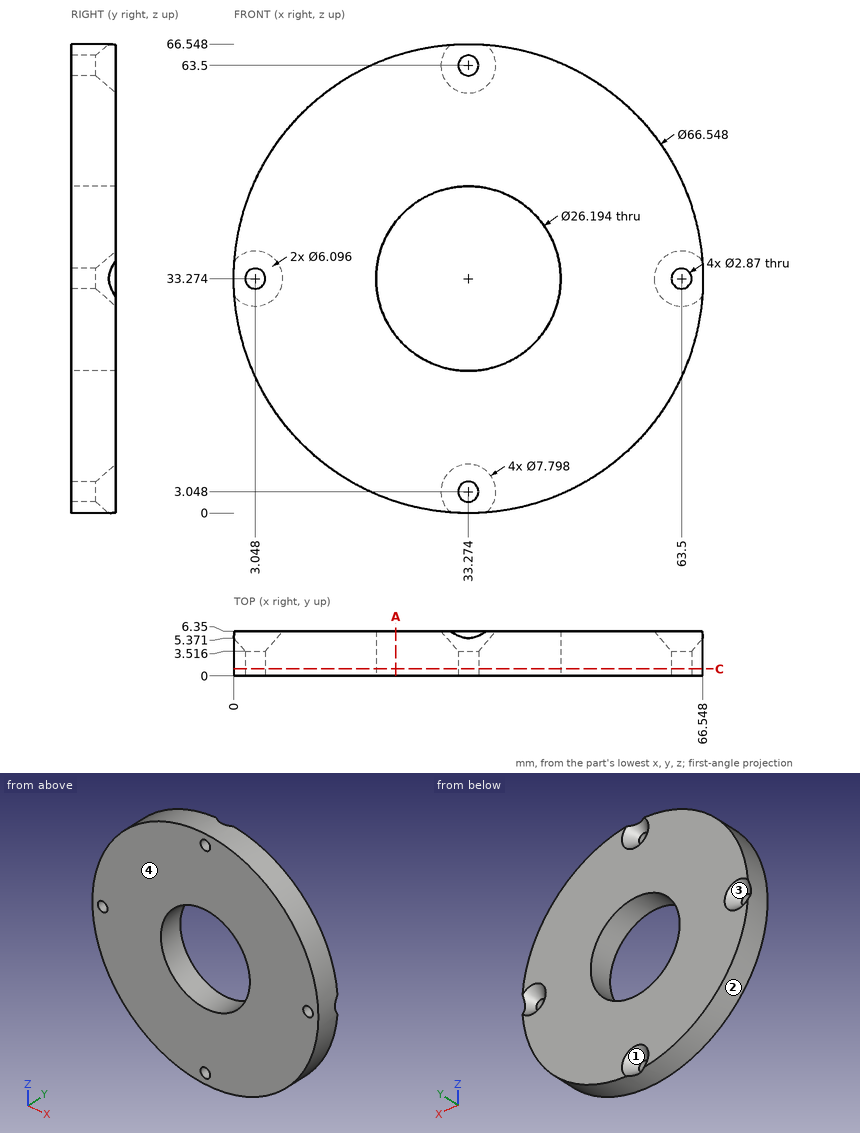
Check sheet for the drawn part. Datum: minimum x, y, z corner. Units: mm. Coordinates: 2 decimals unless noted, no trailing zeros. Write each loop counter-clockwise with the first axis right and the second up, starting at its lowest first coordinate (ties: lowest second). Pieces come first, ordered by that corner, then holes. Notation, with made-up numbers: (21, 62) - (63, 62) arc R33 cw to (63, 95) - close; hole circle Ø9 at (-36, 47.5). An arc over 180 degrees is marked (long way). Answer as a JSON object with one key per item and string values.
(1) Mould release check, pull along Z, two halves, no side actions. Record for the marked faces 1, 2, 3 and 4: pulls with the +Z half, pulls with the -Z half, needs draft (parallel to the pull), parting line crosses it, or undercut.
Report:
{"face 1": "undercut", "face 2": "parting line crosses it", "face 3": "undercut", "face 4": "needs draft"}
(2) Thickness scan on line 1 along Z through (x, y) = (34.5, 4.25) (1 decimal); line 2 along X through (y, z) = (4.5, 62) (1 decimal); line 3 along X through (y, z) = (4.25, 22). Record the ranges inside material, lowest first.
Report:
{"line 1": "0 to 1.4, 4.7 to 20.2, 46.3 to 61.8, 65.2 to 66.5", "line 2": "16.5 to 31.5, 35 to 50.1", "line 3": "1.97 to 26.61, 39.94 to 64.58"}
(3) Cross-section at A-A on x = 23. Record the cut outline in (y, z).
Report:
{"outline": "(0, 1.63) - (6.35, 1.63) - (6.35, 25.15) - (0, 25.15) - close; (0, 41.4) - (6.35, 41.4) - (6.35, 64.92) - (0, 64.92) - close"}
(4) Gauge pin test, flat ends, axial feed: pin 1 Ø1 at (x, y) = (25.5, 0.5) entering from -Z (1 decimal); pin 2 Ø3.5 at (x, z) = (33.274, 3.048) entering from -Y; pin 3 Ø4.5 at (x, z) = (3.048, 33.274) entering from +Y; pin 4 Ø21 at (x, z) = (33.274, 33.274) entering from +Y. Record the tip position at first contact, or that the pin passes through.
Report:
{"pin 1": "z = 0.8", "pin 2": "y = 0", "pin 3": "y = 4.45", "pin 4": "through"}
(5) Cross-section at C-C on y = 1. Record the cut outline in (x, z) (1 decimal).
Report:
{"outline": "circle Ø66.5 at (33.3, 33.3); hole circle Ø2.9 at (3, 33.3); hole circle Ø26.2 at (33.3, 33.3); hole circle Ø2.9 at (33.3, 3); hole circle Ø2.9 at (33.3, 63.5); hole circle Ø2.9 at (63.5, 33.3)"}
